from build123d import *


with BuildPart() as part:
    # 草图1 → 旋转1 (revolve)
    with BuildSketch(Plane.XY, mode=Mode.PRIVATE) as revolve_1_sk:
        with BuildLine():
            Line((9.7, 42.5), (0.6, 42.5))
            ThreePointArc((0.6, 42.5), (0.175735931, 42.324264069), (0, 41.9))
            Line((0, 41.9), (0, 39.25))
            Line((0, 39.25), (2.842505156, 39.25))
            ThreePointArc((2.842505156, 39.25), (4.193041023, 40.158213914), (5.820549028, 40.154050356))
            Line((5.820549028, 40.154050356), (10, 40.3))
            Line((10, 40.3), (10, 42.2))
            ThreePointArc((10, 42.2), (9.912132034, 42.412132034), (9.7, 42.5))
        make_face()
    revolve(revolve_1_sk.sketch.rotate(Axis((-0.001270488, 0, 0), (1, 0, 0)), 270), axis=Axis((-0.001270488, 0, 0), (1, 0, 0)))


solid = part.part
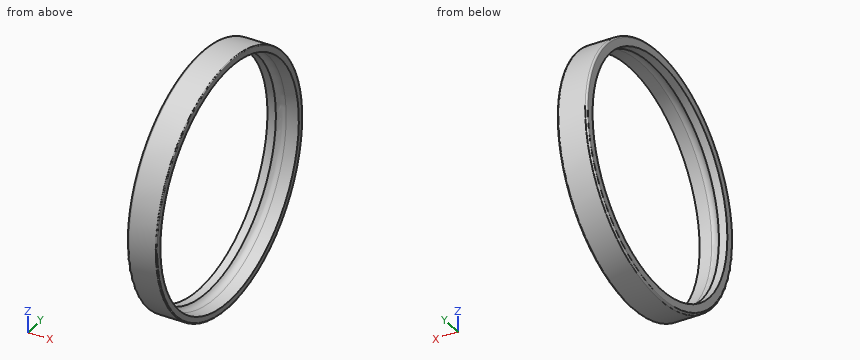
Here's how the part is built. I have some questions about the finished solid (model axes, mm). Coordinates: 2 decimals unless noted, no trailing zeros. Loops run counter-clockwise (first coordinate to the right, second up) from the corner with the lowest first, then second, coordinate; pieces in that order, holes last. Notation, with made-up numbers: (0.25, 78) -> (46.25, 78) arc R24 cw to (46.25, 98) -> close; hole circle Ø3 at (-14, 82). An arc over 180 degrees is marked (long way). Use one line per item in the form item = value. Start each with the question number.
(1) If we section it at A-A (y = 0): Please give me the cut outline in (x, z).
(2) Will these pins go through, and if not, where does the flat tip stop? pin 1 (1.5 mm diameter, centred on x = 3.5, y = 8, fed in from +Z); pin 2 (3 mm diameter, centred on x = 5, z = -23, fed in from -Y); pin 3 (4 mm diameter, centred on x = 9, y = 15.5, fed in from -Z).
(3) Please list where these lines run through material, in increasing order: line 1 along Y through (x, z) = (1.4, 0); line 2 along Y through (x, z) = (7.5, -23); line 3 along Z through (x, y) = (1, 33).
(4) If we section it at C-C (x = 7.75): Please give me the cut outline in (y, z).
Verdict:
q1.outline = (0, -41.9) arc R0.6 ccw to (0.6, -42.5) -> (9.7, -42.5) arc R0.3 ccw to (10, -42.2) -> (10, -40.3) -> (5.82, -40.15) arc R2.78 cw to (2.84, -39.25) -> (0, -39.25) -> close; (0, 39.25) -> (2.84, 39.25) arc R2.78 cw to (5.82, 40.15) -> (10, 40.3) -> (10, 42.2) arc R0.3 ccw to (9.7, 42.5) -> (0.6, 42.5) arc R0.6 ccw to (0, 41.9) -> close
q2.pin_1 = 41.88
q2.pin_2 = -36.66
q2.pin_3 = -40.3
q3.line_1 = -42.5 to -39.25, 39.25 to 42.5
q3.line_2 = -35.74 to -32.99, 32.99 to 35.74
q3.line_3 = -26.78 to -21.25, 21.25 to 26.78
q4.outline = circle Ø85 at (0, 0); hole circle Ø80.44 at (0, 0)
